Source: CAD feature listing. Evaluate the final solid. Frame: model axes, mm. A direction names the side the tool comes from. Round coordinates to 2 decimals unless told otherwise and drop trailing zeros. Write each loop counter-clockwise with the first axis right and the second up, starting at its lowest first coordinate (ties: lowest second). Pieces come first, ordered by that corner, then holes. Notation, with made-up numbers: M 56.5,-2 L 71.5,-2 A18 ccw 71.5,12 Z; hole C 8,-11.5 d3. An arc over 180 degrees is marked long. Use a Markdown table: item, result.
```python
from build123d import *

# Parameters (mm, degrees)
F0_W     = 45
F0_H     = 37
F1_DEPTH = 8
F3_DEPTH = 37.001


with BuildPart() as f1:
    # F0 (on Top) → F1 (new body)
    with BuildSketch(Plane.XY):
        Rectangle(F0_W, F0_H)
    extrude(amount=F1_DEPTH)

    # F2 (on face) → F3 (cut, through all)
    with BuildSketch(Plane.XZ.offset(18.5)):
        Polygon((15.7, 8), (-15.7, 8), (-17.7, 3.392867), (-17.7, 3), (17.7, 3), (17.7, 3.392867), align=None)
    extrude(amount=-F3_DEPTH, mode=Mode.SUBTRACT)


solid = f1.part
```
Q1. Section A-A on z = 6. Return loops of the section in (x, y), plus the area to 3 significant figures.
Results are:
| item | result |
|---|---|
| outline | M -22.5,-18.5 L -16.57,-18.5 L -16.57,18.5 L -22.5,18.5 Z; M 16.57,-18.5 L 22.5,-18.5 L 22.5,18.5 L 16.57,18.5 Z |
| area | 439 mm^2 |
Q2. Mould query, pull axis Z, two halves, no side actions, for faces 1 (the flat face through (19, 0, 8)), 2 (the flat face through (-16.7, -0.3, 5.7)), 3 (the flat face through (0, 0, 0)). Classes: +Z half, -Z half, draft (parallel to the pull), parting line (faces both ways), or undercut.
Results are:
| item | result |
|---|---|
| face 1 | +Z half |
| face 2 | undercut |
| face 3 | -Z half |
Q3. Reachability of faces 4 (the flat face through (-22.5, 0, 4)), 5 (the flat face through (16.7, -0.3, 5.7)) from +Z, -Z, +X, -X, +Y, -Y: full face, straight path, thin tool, end or side. Return the list, or none.
Results are:
| item | result |
|---|---|
| face 4 | +Z, -Z, -X, +Y, -Y |
| face 5 | +Y, -Y |
Q4. Section B-B on y = 9. Return loops of the section in (x, z), plus the area to 3 significant figures.
Results are:
| item | result |
|---|---|
| outline | M -22.5,0 L 22.5,0 L 22.5,8 L 15.7,8 L 17.7,3.39 L 17.7,3 L -17.7,3 L -17.7,3.39 L -15.7,8 L -22.5,8 Z |
| area | 192 mm^2 |
Q5. Section C-C on x = -15. Return loops of the section in (y, z), plus the area to 3 significant figures.
Results are:
| item | result |
|---|---|
| outline | M -18.5,0 L 18.5,0 L 18.5,3 L -18.5,3 Z |
| area | 111 mm^2 |
Q6. Line query: L1, parallel to X at y = -10.5, z = 6; L2, parallel to Z at x = 9, y = 11; L3, parallel to X at y = 15.5, z = 7. Output: solid intervals per line, ascending.
Results are:
| item | result |
|---|---|
| L1 | -22.5 to -16.57, 16.57 to 22.5 |
| L2 | 0 to 3 |
| L3 | -22.5 to -16.13, 16.13 to 22.5 |
Q7. First-contact query: pin 1 Ø2 at (x, y) = (5, 4) entering from +Z. Flat tip, straight axial feed; report the tip coordinate or a pass-through.
Results are:
| item | result |
|---|---|
| pin 1 | z = 3 |
